Geometry check sheet. Reference: the model listing, model coordinates, mm. Coordinates: 2 decimals unless noted, no trailing zeros. Order: outer loops, then holes, each group sorted by start corner. A loop starts at its lowest first (then second) coordinate and runs counter-clockwise, first axis right, second up. Notation, with made-up numbers: (54, 80.5) - (82, 80.5) arc R17 cw to (82, 89.5) - close; hole circle Ø10 at (47, 54). An arc over 180 degrees is marked (long way). Put each result on its own line as item: value.
from build123d import *

# Parameters (mm, degrees)
SKETCH1_W                 = 41.91
SKETCH1_H                 = 57.277
SKETCH1_R                 = 17.653
BOSS_EXTRUDE1_DEPTH       = 6.35
CUT_EXTRUDE1_REACH        = 63.32
CUT_EXTRUDE1_END_RADIUS   = 17.653
SKETCH4_W                 = 1.27
SKETCH4_H                 = 12.7
SKETCH9_R                 = 1.7859375
CUT_EXTRUDE2_DEPTH        = 20.32
F_6_32_TAPPED_HOLE1_D     = 2.7051
F_4_40_TAPPED_HOLE3_D     = 2.2606
F_4_40_TAPPED_HOLE3_DEPTH = 12.7
F_4_40_TAPPED_HOLE3_TIP   = 0.679152758


with BuildPart() as part:
    # Sketch1 → Boss-Extrude1 (new, symmetric)
    with BuildSketch(Plane.XY):
        with Locations((0, 28.6385)):
            Rectangle(SKETCH1_W, SKETCH1_H)
        with Locations((0, 33.274)):
            Circle(SKETCH1_R, mode=Mode.SUBTRACT)
    extrude(amount=BOSS_EXTRUDE1_DEPTH, both=True)

    # Cut-Extrude1: up to this cylinder (the profile starts outside it)
    cut_extrude1_end = Plane(origin=(0, 33.274, 0), z_dir=(0, 0, -1)) * Cylinder(CUT_EXTRUDE1_END_RADIUS, 162.946, mode=Mode.PRIVATE)
    # Sketch4 → Cut-Extrude1 (cut, up to the surface)
    with BuildSketch(Plane(origin=(0, 57.277, 0), x_dir=(1, 0, 0), z_dir=(0, 1, 0)), mode=Mode.PRIVATE) as cut_extrude1_sk1:
        Rectangle(SKETCH4_W, SKETCH4_H)
    cut_extrude1_tool1 = extrude(cut_extrude1_sk1.sketch, amount=-CUT_EXTRUDE1_REACH, mode=Mode.PRIVATE) - cut_extrude1_end
    add(cut_extrude1_tool1.solids().sort_by_distance((0, 57.277, 0))[0], mode=Mode.SUBTRACT)

    # Sketch9 → Cut-Extrude2 (cut)
    with BuildSketch(Plane.ZY.offset(20.955)):
        with Locations(Location((0, 54.09628772, 0), (0, 0, 270))):
            Circle(SKETCH9_R)
    extrude(amount=-CUT_EXTRUDE2_DEPTH, mode=Mode.SUBTRACT)

    # #6-32 Tapped Hole1 (through all)
    with Locations(Plane.ZY.offset(-0.635)):
        with Locations((0, 54.09628772)):
            Hole(F_6_32_TAPPED_HOLE1_D / 2)

    # #4-40 Tapped Hole3
    with Locations(Plane.XZ):
        with Locations((-14.605, 0), (14.605, 0)):
            Hole(F_4_40_TAPPED_HOLE3_D / 2, depth=F_4_40_TAPPED_HOLE3_DEPTH)
            with Locations((0, 0, -(F_4_40_TAPPED_HOLE3_DEPTH + F_4_40_TAPPED_HOLE3_TIP / 2))):  # 118° drill point
                Cone(0, F_4_40_TAPPED_HOLE3_D / 2, F_4_40_TAPPED_HOLE3_TIP, mode=Mode.SUBTRACT)


solid = part.part
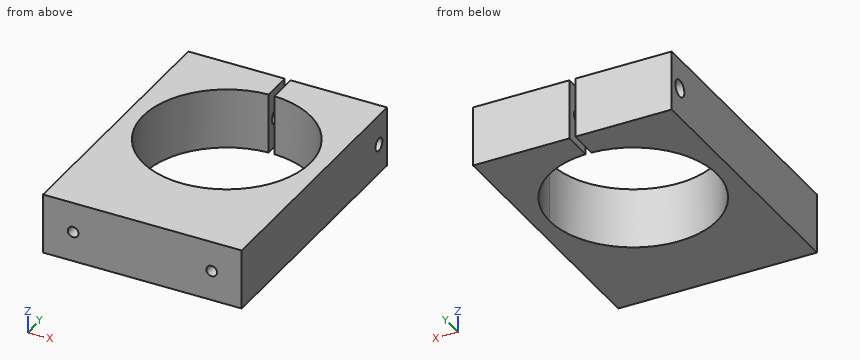
Q1. Depth check by flat-ended pin: pin 1 Ø6 at (x, y) = (-13, 40.5) entering from +Z; pin 2 Ø1.4 at (x, z) = (-14.605, 0) entering from -Y; pin 3 Ø2 at (y, z) = (54.1, 0) entering from +X. Enter the tip coordinate at first touch or a pass-through.
Answer block:
pin 1: stops at z = 6.35
pin 2: stops at y = 12.96
pin 3: passes through
Q2. Section check C-C on z = 4.5. Record the boundary of the cut face in (x, y) (3 decimals), then the cut area to 3 significant figures.
Answer block:
outline: (-20.955, 0) - (20.955, 0) - (20.955, 57.277) - (0.635, 57.277) - (0.635, 50.916) arc R17.653 cw (long way) to (-0.635, 50.916) - (-0.635, 57.277) - (-20.955, 57.277) - close
area: 1,410 mm^2
Q3. Section check D-D on y = 18.5. Record the boundary of the cut face in (x, z) (3 decimals), then the cut area to 3 significant figures.
Answer block:
outline: (-20.955, -6.35) - (-9.662, -6.35) - (-9.662, 6.35) - (-20.955, 6.35) - close; (9.662, -6.35) - (20.955, -6.35) - (20.955, 6.35) - (9.662, 6.35) - close
area: 287 mm^2
Q4. Section check B-B on y = 4. Record the boundary of the cut face in (x, z) (3 decimals).
Answer block:
outline: (-20.955, -6.35) - (20.955, -6.35) - (20.955, 6.35) - (-20.955, 6.35) - close; hole circle Ø2.261 at (-14.605, 0); hole circle Ø2.261 at (14.605, 0)
Q5. Section check A-A on x = -11.5. Record the boundary of the cut face in (y, z), then the cut area to 3 significant figures.
Answer block:
outline: (0, -6.35) - (19.88, -6.35) - (19.88, 6.35) - (0, 6.35) - close; (46.67, -6.35) - (57.28, -6.35) - (57.28, 6.35) - (46.67, 6.35) - close; hole circle Ø3.57 at (54.1, 0)
area: 377 mm^2
Q6. Thickness scan on L1, parallel to X at y = 9.5, z = 0 (3 decimals); L2, parallel to Y at x = 7.5, z = 0; L3, parallel to Y at x = -5.5, z = 1.5. Record the ranges inside material, lowest first. Write a range as [from, to].
Answer block:
L1: x = [-20.955, -15.735], [-13.475, 13.475], [15.735, 20.955]
L2: y = [0, 17.29], [49.25, 52.74], [55.45, 57.28]
L3: y = [0, 16.5], [50.05, 53.13], [55.07, 57.28]
